Check sheet for the modelled part. Datum: model origin and axes. Units: mm. Give positions to 0.01 mm unless a question says otherwise; leave off trailing zeros. Order: outer loops, then holes, each group sorted by start corner. A loop starts at its lowest first (then second) coordinate and runs counter-clockwise, first axis right, second up.
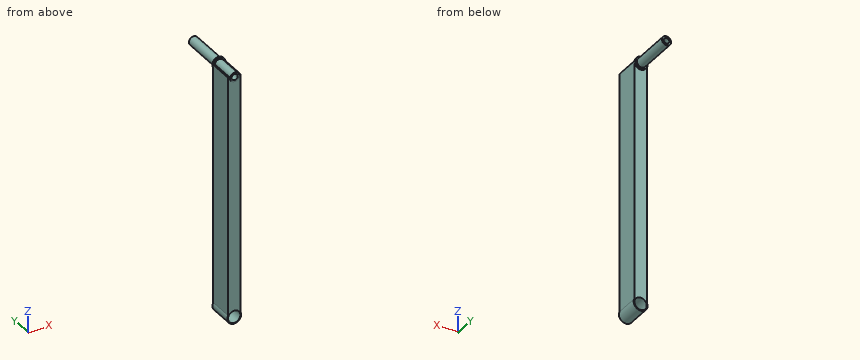
```python
from build123d import *

# Parameters (mm, degrees)
SKETCH1_W                       = 25.4
SKETCH1_H                       = 50.8
SKETCH1_W_2                     = 22.2504
SKETCH1_H_2                     = 47.6504
BOSS_EXTRUDE1_DEPTH             = 498.475
SKETCH2_R                       = 14.2875
SKETCH2_R_2                     = 9.525
CUT_EXTRUDE1_DEPTH              = 51.8
SKETCH3_R                       = 14.2875
SKETCH3_R_2                     = 12.6365
BOSS_EXTRUDE2_DEPTH             = 50.8
SKETCH4_R                       = 9.525
SKETCH4_R_2                     = 6.35
BOSS_EXTRUDE3_DEPTH             = 88.9
BOSS_EXTRUDE3_DEPTH_BACK        = 52.3875
SKETCH5_R                       = 12.7
SKETCH5_R_2                     = 9.525
BOSS_EXTRUDE4_DEPTH             = 3.175
SKETCH6_R                       = 6.35
BOSS_EXTRUDE5_DEPTH             = 19.05
TAP_DRILL_FOR_1_2_20_TAP1_D     = 11.50874
TAP_DRILL_FOR_1_2_20_TAP1_DEPTH = 19.05
BOSS_EXTRUDE6_REACH             = 28.987
SKETCH9_W                       = 1.524
SKETCH9_H                       = 50.8
BOSS_EXTRUDE7_REACH             = 28.988
SKETCH10_W                      = 1.524
SKETCH10_H                      = 50.8


with BuildPart() as part:
    # Sketch1 → Boss-Extrude1 (new body)
    with BuildSketch(Plane.XY):
        Rectangle(SKETCH1_W, SKETCH1_H)
        Rectangle(SKETCH1_W_2, SKETCH1_H_2, mode=Mode.SUBTRACT)
    extrude(amount=BOSS_EXTRUDE1_DEPTH)

    # Sketch2 → Cut-Extrude1 (cut, through all)
    with BuildSketch(Plane(origin=(0, 25.4, 0), x_dir=(1, 0, 0), z_dir=(0, 1, 0))):
        Circle(SKETCH2_R)
        with Locations((0, -498.475)):
            Circle(SKETCH2_R_2)
    extrude(amount=-CUT_EXTRUDE1_DEPTH, mode=Mode.SUBTRACT)

    # Sketch3 → Boss-Extrude2 (add)
    with BuildSketch(Plane(origin=(0, 25.4, 0), x_dir=(1, 0, 0), z_dir=(0, 1, 0))):
        Circle(SKETCH3_R)
        Circle(SKETCH3_R_2, mode=Mode.SUBTRACT)
    extrude(amount=-BOSS_EXTRUDE2_DEPTH)

    # Sketch4 → Boss-Extrude3 (add, two sides)
    with BuildSketch(Plane(origin=(0, 25.4, 0), x_dir=(1, 0, 0), z_dir=(0, 1, 0))) as boss_extrude3_sk:
        with Locations((0, -498.475)):
            Circle(SKETCH4_R)
        with Locations((0, -498.475)):
            Circle(SKETCH4_R_2, mode=Mode.SUBTRACT)
    extrude(amount=BOSS_EXTRUDE3_DEPTH)
    extrude(boss_extrude3_sk.sketch, amount=-BOSS_EXTRUDE3_DEPTH_BACK)

    # Sketch5 → Boss-Extrude4 (add)
    with BuildSketch(Plane(origin=(0, 25.4, 0), x_dir=(1, 0, 0), z_dir=(0, 1, 0))):
        with Locations((0, -498.475)):
            Circle(SKETCH5_R)
        with Locations((0, -498.475)):
            Circle(SKETCH5_R_2, mode=Mode.SUBTRACT)
    extrude(amount=BOSS_EXTRUDE4_DEPTH)

    # Sketch6 → Boss-Extrude5 (add)
    with BuildSketch(Plane(origin=(0, 114.3, 0), x_dir=(1, 0, 0), z_dir=(0, 1, 0))):
        with Locations((0, -498.475)):
            Circle(SKETCH6_R)
    extrude(amount=-BOSS_EXTRUDE5_DEPTH)

    # Tap Drill for 1/2-20 Tap1
    with Locations(Plane(origin=(0, 114.3, 0), x_dir=(1, 0, 0), z_dir=(0, 1, 0))):
        with Locations((0, -498.475)):
            Hole(TAP_DRILL_FOR_1_2_20_TAP1_D / 2, depth=TAP_DRILL_FOR_1_2_20_TAP1_DEPTH)

    # Sketch9 → Boss-Extrude6 (add, up to next)
    with BuildSketch(Plane(origin=(12.7, 0, 0), x_dir=(0, 0, -1), z_dir=(1, 0, 0)), mode=Mode.PRIVATE) as boss_extrude6_sk1:
        with Locations((-499.237, 0)):
            Rectangle(SKETCH9_W, SKETCH9_H)
    boss_extrude6_tool1 = extrude(boss_extrude6_sk1.sketch, amount=-BOSS_EXTRUDE6_REACH, mode=Mode.PRIVATE) - part.part
    add(boss_extrude6_tool1.solids().sort_by_distance((12.7, 0, 499.237))[0])

    # Sketch10 → Boss-Extrude7 (add, up to next)
    with BuildSketch(Plane.ZY.offset(12.7), mode=Mode.PRIVATE) as boss_extrude7_sk1:
        with Locations((499.237, 0)):
            Rectangle(SKETCH10_W, SKETCH10_H)
    boss_extrude7_tool1 = extrude(boss_extrude7_sk1.sketch, amount=-BOSS_EXTRUDE7_REACH, mode=Mode.PRIVATE) - part.part
    add(boss_extrude7_tool1.solids().sort_by_distance((-12.7, 0, 499.237))[0])


solid = part.part
```
(1) Cross-section at B-B on z = 0. Enter the section's corners in (x, y).
Response values:
outline: (-14.29, -25.4) - (-12.64, -25.4) - (-12.64, 25.4) - (-14.29, 25.4) - close; (12.64, -25.4) - (14.29, -25.4) - (14.29, 25.4) - (12.64, 25.4) - close
(2) Gauge pin test, flat ends, axial feed: pin 1 Ø3 at (x, y) = (1, -4.5) entering from +Z; pin 2 Ø3 at (x, y) = (-9, 19) entering from -Z; pin 3 Ø6 at (x, y) = (9.5, 45) entering from +Z; pin 4 Ø7.5 at (x, z) = (0, 498.475) entering from -Y. Record the tip position at first contact, or that the pin passes through.
Response values:
pin 1: stops at z = 508
pin 2: stops at z = -12.16
pin 3: stops at z = 505.44
pin 4: passes through
(3) Cross-section at A-A on x = 0. Count the separate pieces of the cut face and the enclosed holes in it, then the cut area to 3 significant figures.
Response values:
separate pieces: 3
enclosed holes: 1
area: 2,600 mm2
(4) Material ranges on L1, parallel to Y at x = -0.25, z = 164; L2, parallel to Z at x = 0, y = 99; L3, parallel to Z at x = 0, y = 32 (3 decimals), recorded low to high.
Response values:
L1: y = -25.4 to -23.83, 23.83 to 25.4
L2: z = 488.95 to 492.72, 504.23 to 508
L3: z = 488.95 to 492.125, 504.825 to 508
(5) Cross-section at C-C on z = 88. Enter the section's corners in (x, y), then the cut area to 3 significant figures.
Response values:
outline: (-12.7, -25.4) - (12.7, -25.4) - (12.7, 25.4) - (-12.7, 25.4) - close; hole (-11.13, -23.83) - (11.13, -23.83) - (11.13, 23.83) - (-11.13, 23.83) - close
area: 230 mm2
